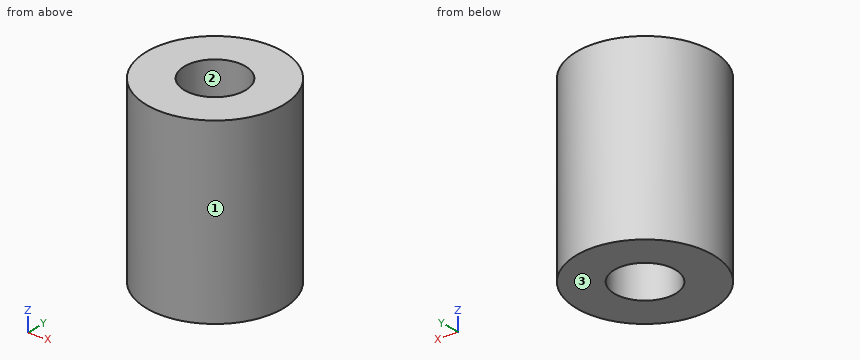
from build123d import *

# Parameters (mm, degrees)
SKETCH1_R           = 9.5
BOSS_EXTRUDE1_DEPTH = 25
SKETCH1_3_R         = 9.5
BOSS_EXTRUDE2_DEPTH = 25
SKETCH2_R           = 4.25
CUT_EXTRUDE1_DEPTH  = 25


with BuildPart() as part:
    # Sketch1 → Boss-Extrude1 (new body)
    with BuildSketch(Plane.XY):
        Circle(SKETCH1_R)
    extrude(amount=BOSS_EXTRUDE1_DEPTH)

    # Sketch1<3> → Boss-Extrude2 (add)
    with BuildSketch(Plane.XY):
        Circle(SKETCH1_3_R)
    extrude(amount=BOSS_EXTRUDE2_DEPTH)

    # Sketch2 → Cut-Extrude1 (cut)
    with BuildSketch(Plane.XY.offset(25)):
        Circle(SKETCH2_R)
    extrude(amount=-CUT_EXTRUDE1_DEPTH, mode=Mode.SUBTRACT)


solid = part.part
Geometry: final body of the model. Coordinates: model frame, mm. Face numbers are marked on the shaded views. Give positions to 0.01 mm unless a question says otherwise; leave off trailing zeros. Write each loop counter-clockwise with the first axis right and the second up, starting at its lowest first coordinate (ties: lowest second). Pieces come first, ordered by that corner, then holes. Notation, with made-up numbers: (87, 21.5) -> (142, 21.5) arc R24 cw to (142, 33.5) -> close; hole circle Ø8 at (87, 82.25). An arc over 180 degrees is marked (long way). Answer as a JSON object with one key per item and string values.
1. Contact query for flat-ended pins moving along their axis: pin 1 (1.5 mm diameter, centred on y = -5.5, z = 17, fed in from -X); pin 2 (8 mm diameter, centred on x = 5.5, z = 14.5, fed in from +Y); pin 3 (10 mm diameter, centred on x = 0, y = 0, fed in from -Z); pin 4 (5 mm diameter, centred on x = -3, z = 21.5, fed in from -Y). Output: stop coordinate, or through.
Ans:
{"pin 1": "stops at x = -8.23", "pin 2": "stops at y = 9.38", "pin 3": "stops at z = 0", "pin 4": "stops at y = -9.49"}
2. Cut plane A-A on y = 0. Output: boundary loops of the cut face in (x, z), and give its area (4 significant figures).
Ans:
{"outline": "(-9.5, 0) -> (-4.25, 0) -> (-4.25, 25) -> (-9.5, 25) -> close; (4.25, 0) -> (9.5, 0) -> (9.5, 25) -> (4.25, 25) -> close", "area": "262.5 mm^2"}
3. Cut plane D-D on y = -5. Output: boundary loops of the cut face in (x, z), and give its area (3 significant figures).
Ans:
{"outline": "(-8.08, 0) -> (8.08, 0) -> (8.08, 25) -> (-8.08, 25) -> close", "area": "404 mm^2"}
4. Mould query, pull axis X, two halves, no side actions, for the marked faces 1, 2 and 3. Classes: pulls with the +X half, pulls with the -X half, needs draft (parallel to the pull), parting line crosses it, or undercut.
Ans:
{"face 1": "parting line crosses it", "face 2": "undercut", "face 3": "needs draft"}
5. Cut plane C-C on z = 16.25. Output: boundary loops of the cut face in (x, y), and give its area (3 significant figures).
Ans:
{"outline": "circle Ø19 at (0, 0); hole circle Ø8.5 at (0, 0)", "area": "227 mm^2"}
6. Ray query, probe 1 along Y at (x, z) = (0, 11); probe 2 along X at (y, z) = (-1.5, 15.5); probe 3 along Y at (x, z) = (-3.5, 4.25). Return the intervals inside material, ascending. Write a range as from..to.
Ans:
{"probe 1": "y = -9.5..-4.25, 4.25..9.5", "probe 2": "x = -9.38..-3.98, 3.98..9.38", "probe 3": "y = -8.83..-2.41, 2.41..8.83"}
